Verification items for the finished model (mm, model axes). Face numbers are marked on the shaded views. A direction names the side the tool comes from. Coordinates: 2 decimals unless noted, no trailing zeros. Loops run counter-clockwise (first coordinate to the right, second up) from the corner with the lowest first, then second, coordinate; pieces in that order, holes last. Notation, with made-up numbers: (15.5, 8) - (62.5, 8) arc R19 cw to (62.5, 31) - close; hole circle Ø3 at (11, 39). An arc over 180 degrees is marked (long way). Answer as CSV lines item,"result". Start each with the question number.
1. Gauge pin test, flat ends, axial feed: P1, Ø1.1, axis at y = 1, z = -0.5, coming from the +X side; P2, Ø1.5, axis at x = 10, y = 1.5, coming from the -Z side. Record the tip position at first contact, or that the pin passes through.
2. Cross-section at A-A (x = 13). Enter the section's corners in (y, z).
3. Material ranges on line 1 (X direction, y = 1.6, z = -0.65); line 2 (Y direction, x = 3.5, z = -0.9), recorded low to high. Write a range as [from, to].
4. Set-up check for the marked faces 1 and 2: record each of +Z, -Z, +X, -X, +Y, -Y from which the full face is reachable in a straight line by a thin tool's end or side.
5. Release check for a two-part mould opening along Y. For the marked faces 3, 4 and 5 record: pulls with the +Y half, pulls with the -Y half, needs draft (parallel to the pull), parting line crosses it, or undercut.
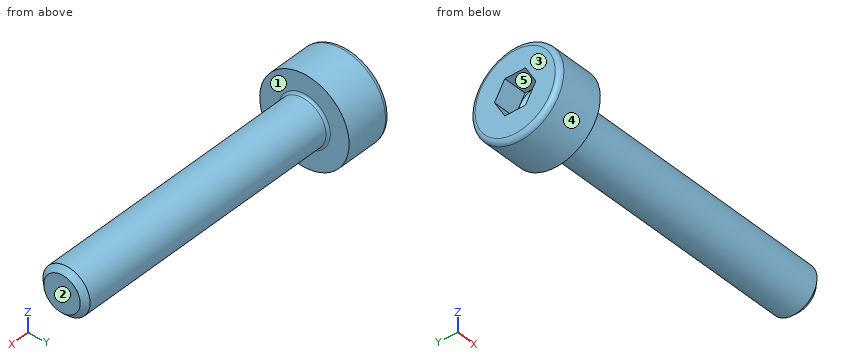
```python
from build123d import *

# Parameters (mm, degrees)
SKETCH_1_W          = 2
SKETCH_1_H          = 1.9
SKETCH_2_R          = 1
EXTRUDE_1_DEPTH     = 12
CUT_EXTRUDE_1_DEPTH = 1
CHAMFER_1_SIZE      = 0.226
FILLET_1_R          = 0.1
FILLET_2_R          = 0.2


with BuildPart() as part:
    # Эскиз1 → Повернуть1 (revolve)
    with BuildSketch(Plane(origin=(0, 0, 0), x_dir=(-1, 0, 0), z_dir=(0, 0, -1)), mode=Mode.PRIVATE) as revolve_1_sk:
        with Locations((-1, 0.95)):
            Rectangle(SKETCH_1_W, SKETCH_1_H)
    revolve(revolve_1_sk.sketch.rotate(Axis((2, 0, 0), (-1, 0, 0)), 270), axis=Axis((2, 0, 0), (-1, 0, 0)))

    # Эскиз2 → Бобышка-Вытянуть1 (add)
    with BuildSketch(Plane(origin=(2, 0, 0), x_dir=(0, 0, -1), z_dir=(1, 0, 0))):
        Circle(SKETCH_2_R)
    extrude(amount=EXTRUDE_1_DEPTH)

    # Эскиз3 → Вырез-Вытянуть1 (cut)
    with BuildSketch(Plane.ZY):
        Polygon((-0.76, -0.438786205), (0, -0.877572409), (0.76, -0.438786205), (0.76, 0.438786205), (0, 0.877572409), (-0.76, 0.438786205), align=None)
    extrude(amount=-CUT_EXTRUDE_1_DEPTH, mode=Mode.SUBTRACT)

    # Эскиз4 → Вырез-Повернуть1 (revolve, cut)
    with BuildSketch(Plane.XY, mode=Mode.PRIVATE) as cut_revolve_1_sk:
        Polygon((1, 0.76), (1, 0), (1.438786205, 0), align=None)
    revolve(cut_revolve_1_sk.sketch.rotate(Axis((0.999975, 0, 0), (1, 0, 0)), 90), axis=Axis((0.999975, 0, 0), (1, 0, 0)), mode=Mode.SUBTRACT)

    # Фаска1
    chamfer_1_edges = [part.edges().sort_by_distance(p)[0] for p in [
        (14, 0, 1),
    ]]
    chamfer(chamfer_1_edges, length=CHAMFER_1_SIZE)

    # Скругление1
    fillet_1_edges = [part.edges().sort_by_distance(p)[0] for p in [
        (2, 0, 1),
    ]]
    fillet(fillet_1_edges, radius=FILLET_1_R)

    # Скругление2
    fillet_2_edges = [part.edges().sort_by_distance(p)[0] for p in [
        (0, 0, -1.9),
    ]]
    fillet(fillet_2_edges, radius=FILLET_2_R)


solid = part.part
```
Values follow:
1,P1,"stops at x = 14"
1,P2,"stops at z = -0.66"
2,outline,"circle Ø2 at (0, 0)"
3,line 1,"x = [0, 2]"
3,line 2,"y = [-0.44, 0.44]"
4,face 1,"+X"
4,face 2,"+Z, -Z, +X, +Y, -Y"
5,face 3,"needs draft"
5,face 4,"parting line crosses it"
5,face 5,"undercut"
